The model under review builds one solid part; all positions refer to its coordinate system, in mm. Face numbers are marked on the shaded views. A direction names the side the tool comes from. Give positions to 0.01 mm unless a question says otherwise; leave off trailing zeros. Order: outer loops, then holes, each group sorted by start corner. A loop starts at its lowest first (then second) coordinate and runs counter-clockwise, first axis right, second up. Notation, with made-up numbers: (-34.5, -1) - (-23.5, -1) arc R8 ccw to (-23.5, 5) - close; hole circle Ø7 at (70.5, 8). An arc over 180 degrees is marked (long way). Use a Markdown table: item, result. Add a question column.
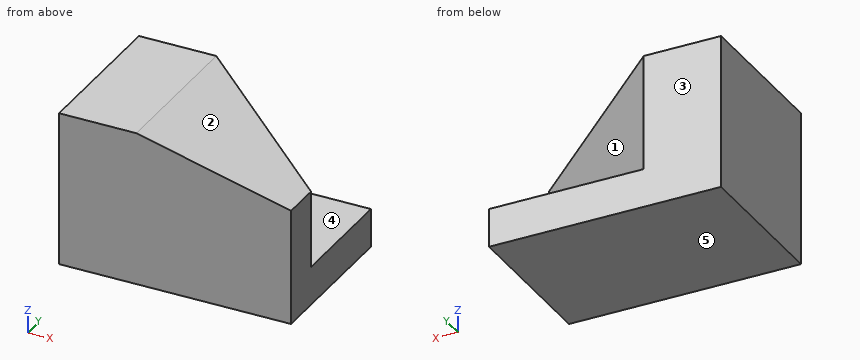
Autodesk Inventor part; units mm, degrees
ref_plane "工作平面1" through (20, 40, 0) normal (-0.6, -0.8, 0) x (0, 0, -1)
ref_plane "YZ Plane" through (0, 0, 0) normal (1, 0, 0) x (0, 1, 0)
ref_plane "XZ Plane" through (0, 0, 0) normal (0, 1, 0) x (-1, 0, 0)
sketch "草圖1" plane through (0, 0, 0) normal (0, 1, 0) x (-1, 0, 0)
  line L0 (0, 0) -> (-60, 0)
  line L1 (-60, 0) -> (-60, -40)
  line L2 (-60, -40) -> (0, -40)
  line L3 (0, -40) -> (0, 0)
  dimension "d0" = 60
  dimension "d1" = 40
extrude "擠出1" add sketch "草圖1" along normal blind 40
sketch "草圖2" plane through (0, 40, 0) normal (0, 1, 0) x (1, 0, 0)
  line L0 (60, 0) -> (60, 40)
  line L1 (60, 0) -> (60, 10)
  line L2 (0, 0) -> (60, 0)
  line L3 (20, 0) -> (60, 0)
  line L4 (20, 0) -> (60, 10)
  dimension "d5" = 20
extrude "擠出2" cut sketch "草圖2" against normal blind 40
sketch "草圖3" plane through (0, 40, 0) normal (0, 1, 0) x (1, 0, 0)
  line L0 (60, 40) -> (0, 40)
  line L1 (0, 40) -> (0, 0)
  line L2 (0, 0) -> (20, 0)
  point P0 (20, 30)
  dimension "d8" = 10
  dimension "d9" = 20
  dimension "d10" = 20
  dimension "d11" = 0
sketch "草圖4" plane through (60, 0, -40) normal (1, 0, 0) x (0, 0, -1)
  line L0 (-30, 40) -> (-30, 0)
  line L1 (-30, 0) -> (0, 0)
  point P0 (-40, 0)
  point P1 (-30, 10)
  dimension "d12" = 10
ref_plane "工作平面1" through (20, 40, 0) normal (-0.6, -0.8, 0) x (0, 0, -1)
sketch "草圖5" plane through (20, 40, 0) normal (-0.6, -0.8, 0) x (0, 0, -1)
  line L0 (-51.3035, -32.4862) -> (51.6467, -32.4862)
  line L1 (51.6467, -32.4862) -> (51.6467, 68.0272)
  line L2 (51.6467, 68.0272) -> (-51.3035, 68.0272)
  line L3 (-51.3035, 68.0272) -> (-51.3035, -32.4862)
  point P0 (0, 8)
extrude "擠出3" cut sketch "草圖5" against normal blind 40
sketch "草圖6" plane through (60, 0, -10) normal (1, 0, 0) x (0, 0, -1)
  line L0 (30, 0) -> (30, 40)
  line L1 (0, 0) -> (30, 0)
  line L2 (30, 0) -> (30, 10)
  line L3 (30, 10) -> (0, 10)
  line L4 (0, 10) -> (0, 0)
  line L5 (30, 0) -> (20, 0)
  line L6 (20, 0) -> (20, 40)
  line L7 (20, 40) -> (30, 40)
  line L8 (30, 40) -> (30, 0)
  line L9 (0, 0) -> (30, 0)
  line L10 (-10, 0) -> (-10, 40)
  dimension "d15" = 10
  dimension "d16" = 10
  dimension "d17" = 0
  dimension "d18" = 10
extrude "擠出4" add sketch "草圖6" against normal up to next
properties part number "50 (74000.000 mm^3)"
Q1. We need section D-D (y = 37). Write out the cut boundary in (x, z).
Q2. We need section B-B (y = 8). Write out the cut boundary in (x, z), plus the area to 3 significant figures.
Q3. We need section C-C (x = 31.5). Write out the cut boundary in (y, z) (1 decimal), plus the area to 3 significant figures.
Q4. Machinability: for the marked faces 1 and 2, which of the approach directions +Z, -Z, +X, -X, +Y, -Y give a long, thin tool a straight path to every point of the face, cutting with its end or side? Answer none if there is none.
Q5. Draft analysis for pull direction Z (two halves, no side actions). For the marked faces 3, 4 and 5, state which applies: pulls with the +Z half, pulls with the -Z half, needs draft (parallel to the pull), parting line crosses it, or undercut.
Q6. Wall thickness on probe 1 along Z at (x, y) = (57.5, 27); probe 2 along X at (y, z) = (19, -21); probe 3 along X at (y, z) = (33.5, -4.5): over which ranges is each line inside the solid? List them lowest first.
Q7. Clearance check with flat-ended pins moving along their axes: P1, Ø3, axis at y = 30.5, z = -15.5, coming from the +X side; P2, Ø10, axis at x = 19, y = 14, coming from the +Z side; P3, Ø24, axis at x = 45.5, y = 17.5, coming from the +Z side (3 decimals). State where each tip first meets the part, or that it passes through.
Here are the results:
| question | item | result |
|---|---|---|
| 1 | outline | (0, -40) - (60, -40) - (60, -30) - (24, -30) - (24, -1) - (20, 0) - (0, 0) - close |
| 2 | outline | (0, -40) - (60, -40) - (60, -10) - (20, 0) - (0, 0) - close |
| 2 | area | 2,200 mm2 |
| 3 | outline | (0, -40) - (40, -40) - (40, -30) - (31.4, -30) - (31.4, -2.9) - (0, -2.9) - close |
| 3 | area | 1,250 mm2 |
| 4 | face 1 | +Z, +X, +Y |
| 4 | face 2 | +Z, +X, +Y, -Y |
| 5 | face 3 | needs draft |
| 5 | face 4 | pulls with the +Z half |
| 5 | face 5 | pulls with the -Z half |
| 6 | probe 1 | -40 to -30 |
| 6 | probe 2 | 0 to 48 |
| 6 | probe 3 | 0 to 28.66 |
| 7 | P1 | x = 34.66 |
| 7 | P2 | z = 0 |
| 7 | P3 | z = -3.375 |
